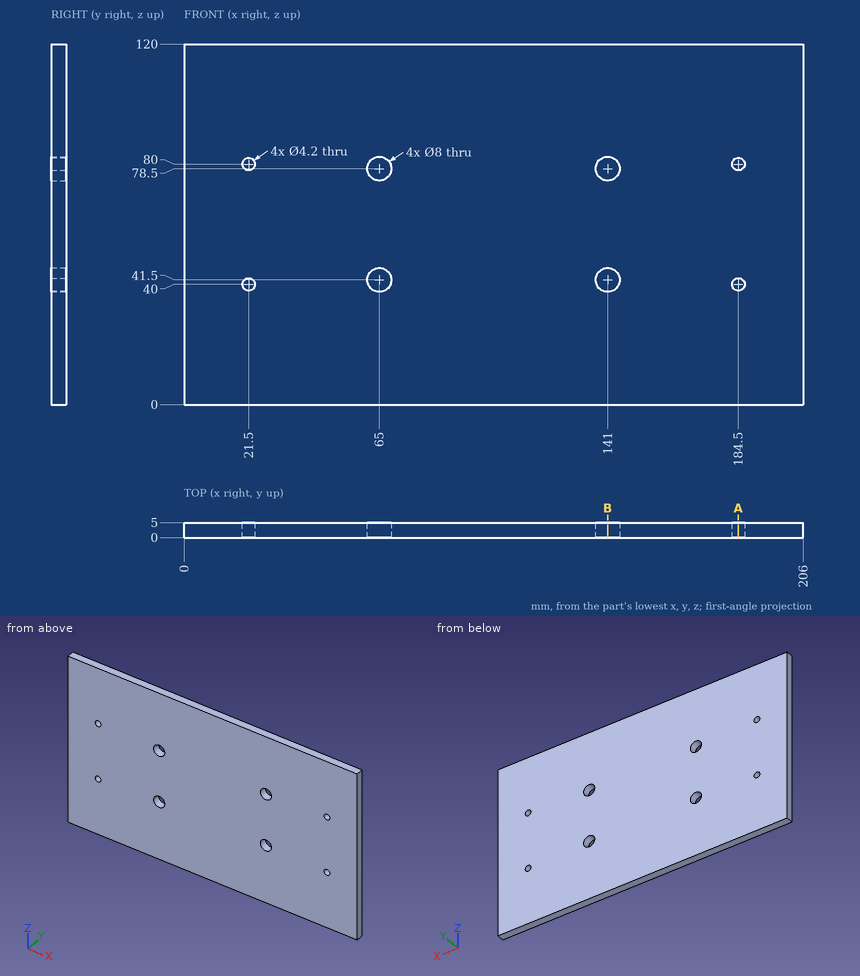
Design review of the part shown in the three views and the two pictorial views. Dimensions are in mm from the part's minimum x, y and z. Round coordinates to 2 decimals unless told otherwise and drop trailing zeros. Loops run counter-clockwise (first coordinate to the right, second up) from the corner with the lowest first, then second, coordinate; pieces in that order, holes last.
Q1. To check wall thickness, follow line 1 along Z through (x, y) = (184.5, 3.95); line 2 along Z through (x, y) = (141, 3.85); line 3 along X through (y, z) = (2.8, 41.5). State the ranges of each line that lie inside material, in increasing order.
Result sheet:
line 1: z = 0 to 37.9, 42.1 to 77.9, 82.1 to 120
line 2: z = 0 to 37.5, 45.5 to 74.5, 82.5 to 120
line 3: x = 0 to 20.03, 22.97 to 61, 69 to 137, 145 to 183.03, 185.97 to 206
Q2. Add section B-B on x = 141. Write out the cut boundary in (y, z).
Result sheet:
outline: (0, 0) - (5, 0) - (5, 37.5) - (0, 37.5) - close; (0, 45.5) - (5, 45.5) - (5, 74.5) - (0, 74.5) - close; (0, 82.5) - (5, 82.5) - (5, 120) - (0, 120) - close
Q3. Insertion check: pin 1 Ø7 at (x, z) = (141, 41.5) entering from +Y. The pin has a flat end and moves straight along its axis. Give the tip position at first contact, or say it passes through.
Result sheet:
pin 1: passes through
Q4. Add section A-A on x = 184.5. Write out the cut boundary in (y, z), plus the area to 3 significant figures.
Result sheet:
outline: (0, 0) - (5, 0) - (5, 37.9) - (0, 37.9) - close; (0, 42.1) - (5, 42.1) - (5, 77.9) - (0, 77.9) - close; (0, 82.1) - (5, 82.1) - (5, 120) - (0, 120) - close
area: 558 mm2
